```python
from build123d import *

# Parameters (mm, degrees)
SKETCH2_R           = 4
CUT_EXTRUDE1_DEPTH  = 9.5
SKETCH3_OUTSIDE_W   = 19.21
SKETCH3_OUTSIDE_H   = 16.456
SKETCH3_OUTSIDE_W_2 = 16.89881261
SKETCH3_OUTSIDE_H_2 = 8.027852412
CUT_EXTRUDE2_DEPTH  = 9.5


with BuildPart() as part:
    # Sketch1 → Revolve4 (revolve)
    with BuildSketch(Plane.XY):
        with BuildLine():
            Line((0, 6.5), (0, -6.5))
            ThreePointArc((0, -6.5), (6.5, 0), (0, 6.5))
        make_face()
    revolve(axis=Axis((0, 0, 0), (0, 1, 0)))

    # Sketch2 → Cut-Extrude1 (cut, symmetric)
    with BuildSketch(Plane(origin=(0, 0, 0), x_dir=(1, 0, 0), z_dir=(0, 1, 0))):
        with Locations(Location((0, 0, 0), (0, 0, 180))):
            Circle(SKETCH2_R)
    extrude(amount=CUT_EXTRUDE1_DEPTH, both=True, mode=Mode.SUBTRACT)

    # Sketch3 outside → Cut-Extrude2 (cut, symmetric)
    with BuildSketch(Plane.XY):
        Rectangle(SKETCH3_OUTSIDE_W, SKETCH3_OUTSIDE_H)
        Rectangle(SKETCH3_OUTSIDE_W_2, SKETCH3_OUTSIDE_H_2, mode=Mode.SUBTRACT)
    extrude(amount=CUT_EXTRUDE2_DEPTH, both=True, mode=Mode.SUBTRACT)


solid = part.part
```
Part model, mm, in its own coordinate system. Give positions to 0.01 mm unless a question says otherwise; leave off trailing zeros. Write each loop counter-clockwise with the first axis right and the second up, starting at its lowest first coordinate (ties: lowest second). Pieces come first, ordered by that corner, then holes. Notation, with made-up numbers: (3, 74.25) -> (10, 74.25) arc R27 cw to (10, 100.25) -> close; hole circle Ø9 at (27.5, 42.25). An arc over 180 degrees is marked (long way). Put each result on its own line as item: value. Start each with the question number.
Item 1: Cut at B-B (z = 0). List the corners of the cut face in (x, y).
Item 2: Pull direction X, two halves, no side cores. Call faces 1 (the face through (0.867, 0.056, -3.905)), 2 (the face through (-3, -4.014, -3)): pulls with the +X half, pulls with the -X half, needs draft (parallel to the pull), parting line crosses it, or undercut.
Item 3: Cut at D-D (x = 4.25). List the corners of the cut face in (y, z), then the cut area to 3 significant figures.
Item 4: Cut at C-C (y = 0). List the corners of the cut face in (x, z).
Item 5: Wall check: L1, parallel to Z at x = 0, y = 2; L2, parallel to Z at x = 0, y = 3; L3, parallel to X at y = 0.75, z = 2.5. Give the ranges that are in metal, low to high. Write a range as [from, to].
Item 6: Pin check, flat tips, straight feed: pin 1 Ø4 at (x, y) = (2.5, 2) entering from -Z; pin 2 Ø4 at (x, y) = (5, -0.5) entering from -Z. Stop position of each tip, or through.
Item 7: Cut at A-A (x = 0). List the corners of the cut face in (y, z).
Answer list:
1. outline: (-5.11, -4.01) -> (-4, -4.01) -> (-4, 4.01) -> (-5.11, 4.01) arc R6.5 ccw to start; (4, -4.01) -> (5.11, -4.01) arc R6.5 ccw to (5.11, 4.01) -> (4, 4.01) -> close
2. face 1: undercut
2. face 2: needs draft
3. outline: (-4.01, -2.84) arc R4.92 ccw to (4.01, -2.84) -> (4.01, 2.84) arc R4.92 ccw to (-4.01, 2.84) -> close
3. area: 69.0 mm2
4. outline: circle Ø13 at (0, 0); hole circle Ø8 at (0, 0)
5. L1: z = [-6.18, -4], [4, 6.18]
5. L2: z = [-5.77, -4], [4, 5.77]
5. L3: x = [-5.95, -3.12], [3.12, 5.95]
6. pin 1: stops at z = -6.39
6. pin 2: stops at z = -5.75
7. outline: (-4.01, -5.11) arc R6.5 ccw to (4.01, -5.11) -> (4.01, -4) -> (-4.01, -4) -> close; (-4.01, 4) -> (4.01, 4) -> (4.01, 5.11) arc R6.5 ccw to (-4.01, 5.11) -> close
